The model under review builds one solid part; all positions refer to its coordinate system, in mm. A direction names the side the tool comes from. Coordinates: 2 decimals unless noted, no trailing zeros. Write each loop counter-clockwise with the first axis right and the second up, starting at its lowest first coordinate (ties: lowest second). Pieces come first, ordered by that corner, then holes. Notation, with made-up numbers: (-39.5, -37.5) - (-25.5, -37.5) arc R27 ccw to (-25.5, -11.5) - close; hole circle Ø2 at (67, 79). An arc over 180 degrees is marked (long way). Return JSON: item names as keys, results as strings. Group by question number.
(1) For pin 1 Ø12 at (x, y) = (5.5, -0.5) entering from -Z; pin 2 Ø2.5 at (x, z) = (15, 5.5) entering from -Y; pin 3 Ø4 at (x, z) = (1.5, 8.5) entering from -Y; pin 4 Ø2 at (y, z) = (13, 6.5) entering from +X, all flat-tipped, find the tip position at first contact; note any pin that passes through.
(2) Draft analysis for pull direction X (two halves, no side actions). For faces 1 (the face through (16.87, 2.1, 8.48)), 2 (the face through (-3.902, -17.572, 3.451)), 3 (the face through (16.1, 2.1, 1)), state which applies: released by +X, released by -X, zero draft, split by the parting line, or undercut.
(3) We need section C-C on x = 0. State the section outline as (y, z) points, then the cut area to 3 significant figures.
(4) We need section A-A on y = 0. State the section outline as (x, z) points.
(5) To check wall thickness, follow L1, parallel to Y at x = 0, z = 6.25; L2, parallel to X at y = 0, z = 5.75; L3, parallel to Z at x = 9.5, y = -12. State the ranges of each line that lie inside material, in increasing order. Write a range as from..to.
(6) We need section D-D on z = 3.75. State the section outline as (x, y) points, then the cut area to 3 significant figures.
(7) We need section B-B on z = 8.25. State the section outline as (x, y) points, then the cut area to 3 significant figures.
(8) Tool access review of faces 4 (the face through (16, -5, 4)), 5 (the face through (0, 17, 1)), 6 (the face through (-16.2, 2.1, 1)), 7 (the face through (0, -3, 0.8)): name each direction out of +Z, -Z, +X, -X, +Y, -Y from which nothing blocks a thin tool from reaching the whole face with its end or side.
```python
from build123d import *

# Parameters (mm, degrees)
BOX_W             = 20
BOX_H             = 14
BOX_DEPTH         = 10
BOX001_W          = 44
BOX001_H          = 14
BOX001_DEPTH      = 10
CYLINDER_R        = 18
CYLINDER_DEPTH    = 0.8
CYLINDER002_R     = 16
CYLINDER002_DEPTH = 11
CYLINDER001_R     = 18
CYLINDER001_DEPTH = 10
CYLINDER003_R     = 17
CYLINDER003_DEPTH = 5
CYLINDER004_R     = 2
CYLINDER004_DEPTH = 10


with BuildPart() as cube:
    # Box → Box (new body)
    with BuildSketch(Plane(origin=(-10, 8, 1), x_dir=(1, 0, 0), z_dir=(0, 0, 1))):
        with Locations((10, 7)):
            Rectangle(BOX_W, BOX_H)
    extrude(amount=BOX_DEPTH)


with BuildPart() as cuts:
    # Box001 → Box001 (new body)
    with BuildSketch(Plane(origin=(-22, -5, 1), x_dir=(1, 0, 0), z_dir=(0, 0, 1))):
        with Locations((22, 7)):
            Rectangle(BOX001_W, BOX001_H)
    extrude(amount=BOX001_DEPTH)

    # Fusion: union Cube
    add(cube.part)


with BuildPart() as top:
    # Cylinder → Cylinder (new body)
    with BuildSketch(Plane.XY):
        Circle(CYLINDER_R)
    extrude(amount=CYLINDER_DEPTH)


with BuildPart() as hole:
    # Cylinder002 → Cylinder002 (new body)
    with BuildSketch(Plane.XY):
        Circle(CYLINDER002_R)
    extrude(amount=CYLINDER002_DEPTH)


with BuildPart() as cut001:
    # Cylinder001 → Cylinder001 (new body)
    with BuildSketch(Plane.XY):
        Circle(CYLINDER001_R)
    extrude(amount=CYLINDER001_DEPTH)

    # Cut: cut hole
    add(hole.part, mode=Mode.SUBTRACT)

    # Fusion001: union top
    add(top.part)

    # Cut001: cut cuts
    add(cuts.part, mode=Mode.SUBTRACT)


with BuildPart() as hole001:
    # Cylinder003 → Cylinder003 (new body)
    with BuildSketch(Plane.XY.offset(7)):
        Circle(CYLINDER003_R)
    extrude(amount=CYLINDER003_DEPTH)


with BuildPart() as cut002:
    # Cone → Cone (revolve)
    with BuildSketch(Plane(origin=(0, 0, 7), x_dir=(1, 0, 0), z_dir=(0, -1, 0))):
        Polygon((0, 0), (18, 0), (21, 3), (0, 3), align=None)
    revolve(axis=Axis((0, 0, 7), (0, 0, 1)))

    # Cut002: cut hole001
    add(hole001.part, mode=Mode.SUBTRACT)


with BuildPart() as fusion002:
    # Cylinder004 → Cylinder004 (new body)
    with BuildSketch(Plane.XY):
        Circle(CYLINDER004_R)
    extrude(amount=CYLINDER004_DEPTH)

    # Fusion002: union Cut001, Cut002
    add(cut001.part)
    add(cut002.part)


solid = fusion002.part
```
Ans:
{
 "1": {"pin 1": "z = 0", "pin 2": "y = -11.62", "pin 3": "y = -21", "pin 4": "x = 13.46"},
 "2": {"face 1": "undercut", "face 2": "split by the parting line", "face 3": "zero draft"},
 "3": {"outline": "(-21, 10) - (-18, 7) - (-18, 0) - (18, 0) - (18, 1) - (16, 1) - (16, 0.8) - (2, 0.8) - (2, 10) - (-2, 10) - (-2, 0.8) - (-16, 0.8) - (-16, 10) - close; (17, 7) - (18, 7) - (21, 10) - (17, 10) - close", "area": "96.4 mm²"},
 "4": {"outline": "(-21, 10) - (-18, 7) - (-17, 7) - (-17, 10) - close; (-18, 0) - (18, 0) - (18, 1) - (16, 1) - (16, 0.8) - (2, 0.8) - (2, 10) - (-2, 10) - (-2, 0.8) - (-16, 0.8) - (-16, 1) - (-18, 1) - close; (17, 7) - (18, 7) - (21, 10) - (17, 10) - close"},
 "5": {"L1": "-18..-16, -2..2", "L2": "-2..2", "L3": "0..0.8"},
 "6": {"outline": "(-17.29, -5) arc R18 ccw to (17.29, -5) - (15.2, -5) arc R16 cw to (-15.2, -5) - close; (-15.59, 9) - (-13.23, 9) arc R16 cw to (-10, 12.49) - (-10, 14.97) arc R18 ccw to start; circle Ø4 at (0, 0); (10, 12.49) arc R16 cw to (13.23, 9) - (15.59, 9) arc R18 ccw to (10, 14.97) - close", "area": "125 mm²"},
 "7": {"outline": "circle Ø38.5 at (0, 0); circle Ø4 at (0, 0); hole (-16.25, -5) - (-15.2, -5) arc R16 ccw to (15.2, -5) - (16.25, -5) arc R17 ccw to (14.42, 9) - (13.23, 9) arc R16 ccw to (10, 12.49) - (10, 13.75) arc R17 ccw to (-10, 13.75) - (-10, 12.49) arc R16 ccw to (-13.23, 9) - (-14.42, 9) arc R17 ccw to start", "area": "322 mm²"},
 "8": {"face 4": "none", "face 5": "+Y", "face 6": "-X", "face 7": "+Z"}
}
